Source: CAD feature listing. Evaluate the final solid. Frame: model axes, mm. A direction names the side the tool comes from. Round coordinates to 2 decimals unless told otherwise and drop trailing zeros. Order: outer loops, then holes, each group sorted by start corner. A loop starts at its lowest first (then second) coordinate and runs counter-clockwise, first axis right, second up. Notation, with made-up numbers: (-24, 70) -> (-8, 70) arc R18 ccw to (-8, 83) -> close; hole circle Ø9 at (72.5, 82). An arc over 180 degrees is marked (long way). Write item = value, one per line. Start each with the question number.
(1) Cut plane C-C on x = -9. Return the cut outline in (y, z).
(2) Cut plane B-B on y = 20.75. Return the cut outline in (x, z).
(3) Draft query along Z for faces 1 (the face through (0, 13, -27.1)), 2 (the face through (1, 26, -26)), 3 (the face through (-42.9, 7, 24)). Return one class per face: released by +Z, released by -Z, zero draft, split by the parting line, or undercut.
(4) Contact query for flat-ended pins moving along their axis: pin 1 Ø5 at (y, z) = (8, 21.5) entering from -X; pin 2 Ø1.5 at (x, z) = (46.5, -23) entering from +Y; pin 3 Ø12 at (y, z) = (10, 5.5) entering from -X. Output: stop coordinate, or through.
(5) Ray query, line 1 (X direction, y = 0.6, z = -22.1); line 2 (Z direction, x = 14, y = 18); line 3 (Y direction, x = 20, z = 19). Return the intervals inside material, ascending.
(6) Cut plane A-A on x = 51. Return the cut outline in (y, z), then the cut area to 3 significant figures.
(7) Reachability of faces 4 (the face through (-49.61, 0.99, -21.21)), 5 (the face through (46, 12, 23)), 6 (the face through (-42.9, 7, -24)) from +Z, -Z, +X, -X, +Y, -Y: full face, straight path, thin tool, end or side. Return the list, or none.
from build123d import *

# Parameters (mm, degrees)
SKETCH_1_W          = 112
SKETCH_1_H          = 54.2
SKETCH_1_W_2        = 108
SKETCH_1_H_2        = 50.2
EXTRUDE_1_DEPTH     = 26
SKETCH_2_W          = 108
SKETCH_2_H          = 50.2
SKETCH_2_R          = 1.65
EXTRUDE_2_DEPTH     = 2
EXTRUDE_3_DEPTH     = 10
SKETCH_9_R          = 3.5
SKETCH_9_W          = 20
SKETCH_9_H          = 10
CUT_EXTRUDE_2_DEPTH = 2
FILLET_2_R          = 2
SKETCH_10_W         = 54.2
SKETCH_10_H         = 26
CUT_EXTRUDE_3_DEPTH = 2
FILLET_3_R          = 1


with BuildPart() as part:
    # 草图1 → 凸台-拉伸1 (new body)
    with BuildSketch(Plane(origin=(0, 0, 0), x_dir=(1, 0, 0), z_dir=(0, 1, 0))):
        Rectangle(SKETCH_1_W, SKETCH_1_H)
        Rectangle(SKETCH_1_W_2, SKETCH_1_H_2, mode=Mode.SUBTRACT)
    extrude(amount=EXTRUDE_1_DEPTH)

    # 草图2 → 凸台-拉伸2 (add)
    with BuildSketch(Plane(origin=(0, 0, 0), x_dir=(1, 0, 0), z_dir=(0, 1, 0))):
        Rectangle(SKETCH_2_W, SKETCH_2_H)
        with Locations(Location((-51, 22.1, 0), (0, 0, 270))):
            Circle(SKETCH_2_R, mode=Mode.SUBTRACT)
        with Locations(Location((51, 22.1, 0), (0, 0, 90))):
            Circle(SKETCH_2_R, mode=Mode.SUBTRACT)
        with Locations(Location((51, -22.1, 0), (0, 0, 270))):
            Circle(SKETCH_2_R, mode=Mode.SUBTRACT)
        with Locations(Location((-51, -22.1, 0), (0, 0, 90))):
            Circle(SKETCH_2_R, mode=Mode.SUBTRACT)
    extrude(amount=EXTRUDE_2_DEPTH)

    # 草图6 → 凸台-拉伸3 (add)
    with BuildSketch(Plane(origin=(0, 2, 0), x_dir=(1, 0, 0), z_dir=(0, 1, 0))):
        Polygon((-47.9, 25.1), (-47.9, 19.1), (-46.5, 19.1), (-46.5, 22.1), (-42.9, 22.1), (-42.9, 25.1), align=None)
        Polygon((46.5, 19.1), (46.5, 22.1), (42.9, 22.1), (42.9, 25.1), (47.9, 25.1), (47.9, 19.1), align=None)
        Polygon((47.9, -25.1), (47.9, -19.1), (46.5, -19.1), (46.5, -22.1), (42.9, -22.1), (42.9, -25.1), align=None)
        Polygon((-42.9, -25.1), (-47.9, -25.1), (-47.9, -19.1), (-46.5, -19.1), (-46.5, -22.1), (-42.9, -22.1), align=None)
    extrude(amount=EXTRUDE_3_DEPTH)

    # 草图9 → 切除-拉伸2 (cut)
    with BuildSketch(Plane.ZY.offset(56)):
        with Locations((-16, 6)):
            Circle(SKETCH_9_R)
        with Locations((10.1, 16)):
            Rectangle(SKETCH_9_W, SKETCH_9_H)
    extrude(amount=-CUT_EXTRUDE_2_DEPTH, mode=Mode.SUBTRACT)

    # 圆角2
    fillet_2_edges = [part.edges().sort_by_distance(p)[0] for p in [
        (-56, 16, 20.1),
        (-56, 21, 10.1),
        (-56, 16, 0.1),
        (-56, 11, 10.1),
        (-56, 6, -19.5),
    ]]
    fillet(fillet_2_edges, radius=FILLET_2_R - 0.0001)  # a hair under: the kernel refuses the full size

    # 草图10 → 切除-拉伸3 (cut)
    with BuildSketch(Plane.ZY.offset(56)):
        with Locations((0, 13)):
            Rectangle(SKETCH_10_W, SKETCH_10_H)
    extrude(amount=-CUT_EXTRUDE_3_DEPTH, mode=Mode.SUBTRACT)

    # 圆角3
    fillet_3_edges = [part.edges().sort_by_distance(p)[0] for p in [
        (-42.9, 7, 22.1),
        (-46.5, 7, 22.1),
        (-46.5, 7, 19.1),
        (-46.5, 7, -19.1),
        (-46.5, 7, -22.1),
        (-42.9, 7, -22.1),
        (42.9, 7, -22.1),
        (46.5, 7, -22.1),
        (46.5, 7, -19.1),
        (46.5, 7, 19.1),
        (46.5, 7, 22.1),
        (42.9, 7, 22.1),
    ]]
    fillet(fillet_3_edges, radius=FILLET_3_R)


solid = part.part
Evaluation:
q1.outline = (0, -27.1) -> (26, -27.1) -> (26, -25.1) -> (2, -25.1) -> (2, 25.1) -> (26, 25.1) -> (26, 27.1) -> (0, 27.1) -> close
q2.outline = (-54, -27.1) -> (56, -27.1) -> (56, 27.1) -> (-54, 27.1) -> (-54, 25.1) -> (54, 25.1) -> (54, -25.1) -> (-54, -25.1) -> close
q3.face_1 = released by -Z
q3.face_2 = zero draft
q3.face_3 = undercut
q4.pin_1 = -47.9
q4.pin_2 = 12
q4.pin_3 = 54
q5.line_1 = -54 to -52.65, -49.35 to 49.35, 52.65 to 56
q5.line_2 = -27.1 to -25.1, 25.1 to 27.1
q5.line_3 = 0 to 2
q6.outline = (0, -27.1) -> (26, -27.1) -> (26, -25.1) -> (2, -25.1) -> (2, -23.75) -> (0, -23.75) -> close; (0, -20.45) -> (2, -20.45) -> (2, 20.45) -> (0, 20.45) -> close; (0, 23.75) -> (2, 23.75) -> (2, 25.1) -> (26, 25.1) -> (26, 27.1) -> (0, 27.1) -> close
q6.area = 191 mm^2
q7.face_4 = +Y, -Y
q7.face_5 = -X, +Y
q7.face_6 = +Y
